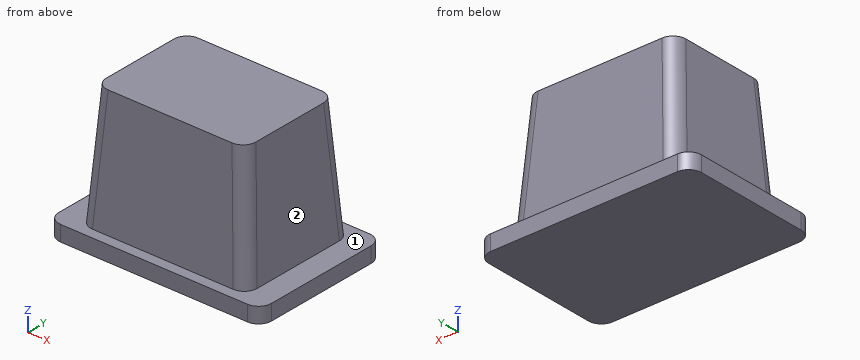
from build123d import *

# Parameters (mm, degrees)
SKETCH1_W           = 130
SKETCH1_H           = 95
BOSS_EXTRUDE1_DEPTH = 100
BOSS_EXTRUDE1_TAPER = 4
SKETCH2_W           = 165
SKETCH2_H           = 110
BOSS_EXTRUDE2_DEPTH = 6
FILLET1_R           = 10
FILLET2_R           = 10


with BuildPart() as part:
    # Sketch1 → Boss-Extrude1 (new body)
    with BuildSketch(Plane.XY):
        with Locations((-26.218487395, 19.642857143)):
            Rectangle(SKETCH1_W, SKETCH1_H)
    extrude(amount=BOSS_EXTRUDE1_DEPTH, taper=BOSS_EXTRUDE1_TAPER)

    # Sketch2 → Boss-Extrude2 (add, symmetric)
    with BuildSketch(Plane.XY):
        with Locations((-26.218487395, 19.642857143)):
            Rectangle(SKETCH2_W, SKETCH2_H)
    extrude(amount=BOSS_EXTRUDE2_DEPTH, both=True)

    # Fillet1
    fillet1_edges = [part.edges().sort_by_distance(p)[0] for p in [
        (-87.512366362, 63.43673611, 53),
        (35.075391572, 63.43673611, 53),
        (35.075391572, -24.151021824, 53),
        (-87.512366362, -24.151021824, 53),
    ]]
    fillet(fillet1_edges, radius=FILLET1_R)

    # Fillet2
    fillet2_edges = [part.edges().sort_by_distance(p)[0] for p in [
        (56.281512605, -35.357142857, 0),
        (56.281512605, 74.642857143, 0),
        (-108.718487395, 74.642857143, 0),
        (-108.718487395, -35.357142857, 0),
    ]]
    fillet(fillet2_edges, radius=FILLET2_R)


solid = part.part
The listing builds one solid part. Answer for the finished solid, in the listing's coordinates (mm). Face numbers are marked on the shaded views. A direction names the side the tool comes from. Coordinates: 2 decimals unless noted, no trailing zeros. Loops run counter-clockwise (first coordinate to the right, second up) from the corner with the lowest first, then second, coordinate; pieces in that order, holes last. Notation, with made-up numbers: (49.25, 56) -> (91.25, 56) arc R23 cw to (91.25, 84) -> close; hole circle Ø11 at (-7.5, 57). An arc over 180 degrees is marked (long way). Answer in a Markdown table with one row per item. Add a question column.
1. Flat-ended cylindrical pins translate along their axes: P1, Ø10, axis at y = 50.5, z = 65, coming from the -X side; P2, Ø6, axis at y = 33.5, z = 41, coming from the -X side; P3, Ø8, axis at y = 51, z = 21, coming from the -X side. Find the tip coordinate at first contact, or state that the pin passes through.
2. The part is cut by section B-B, the plane y = -3. Write down the section's boundary in (x, z).
3. The part is cut by section A-A, the plane x = -23.5. Write down the section's boundary in (y, z), then the cut area to 3 significant figures.
4. Consider line 1 (Z direction, x = -98, y = 15.5); line 2 (Y direction, x = 31.5, z = 91.5); line 3 (X direction, y = 54.5, z = 71). Determine where each line is inside the solid, lowest interval first. Write a range as [from, to].
5. For the marked faces 1 and 2, determine the directions among +Z, -Z, +X, -X, +Y, -Y from which every point of the face is accessible in a straight line to the end or side of a thin tool.
Answer below:
| question | item | result |
|---|---|---|
| 1 | P1 | x = -87.02 |
| 1 | P2 | x = -88.56 |
| 1 | P3 | x = -90.03 |
| 2 | outline | (-108.72, -6) -> (56.28, -6) -> (56.28, 6) -> (38.36, 6) -> (31.79, 100) -> (-84.23, 100) -> (-90.8, 6) -> (-108.72, 6) -> close |
| 3 | outline | (-35.36, -6) -> (74.64, -6) -> (74.64, 6) -> (66.72, 6) -> (60.15, 100) -> (-20.86, 100) -> (-27.44, 6) -> (-35.36, 6) -> close |
| 3 | area | 9,550 mm2 |
| 4 | line 1 | [-6, 6] |
| 4 | line 2 | [-15.59, 54.88] |
| 4 | line 3 | [-85.99, 33.55] |
| 5 | face 1 | +Z |
| 5 | face 2 | +Z, +X, +Y, -Y |
